Source: CAD feature listing. Evaluate the final solid. Frame: model axes, mm. A direction names the side the tool comes from. Give positions to 0.01 mm unless a question says otherwise; leave off trailing zeros. Order: outer loops, then holes, each group sorted by start corner. A loop starts at its lowest first (then second) coordinate and runs counter-clockwise, first axis right, second up.
1) Section C-C, the plane x = -58. Return loops of the section in (y, z), plus the area to 3 significant figures.
2) Material intervals for line 1 (X direction, y = -17, z = 10.5); line 2 (X direction, y = -42, z = 10); line 3 (Y direction, x = 26, z = 1), sorted ascending.
3) Section A-A, the plane z = 6.35. Give the number of separate pieces and of enclosed holes in the cut face, plus the area to 3 significant figures.
4) Section B-B, the plane y = -6. Return loops of the section in (x, z), plus the area to 3 significant figures.
5) Access query for faces 5 (the face through (-68.885, -16, 6)), 6 (the face through (-62.535, -23, 6)), 7 (the face through (81.585, -43, 6)). Directions: +Z, -Z, +X, -X, +Y, -Y. A direction counts if a zero-diameter tool reaches every point of the face in a straight line with its end or side. Return the directions, or none.
6) First-contact query: P1, Ø6.5, axis at y = -32.5, z = 6, coming from the +X side; P2, Ø4, axis at x = 16, z = 7, coming from the -Y side; P3, Ø4, axis at x = -76, z = 5, coming from the +Y side. Flat tips, straight axial feed; report the tip coordinate or a pass-through.
7) Draft query along X for faces 1 (the face through (-1, 0, 6)), 2 (the face through (76.1, -38.608, 4.8)), 3 (the face through (68.885, -16, 6)), 4 (the face through (73.77, -41.74, 5.74)). Return one class per face: released by +X, released by -X, zero draft, split by the parting line, or undercut.
```python
from build123d import *

# Parameters (mm, degrees)
F1_DEPTH = 12.7
F3_R     = 1.5875
F4_DEPTH = 25.4
F2_R     = 1.5875
F5_DEPTH = 25.4
F6_R     = 2.54
F7_R     = 1.778


with BuildPart() as f1:
    # F0 (on Top) → F1 (new body)
    with BuildSketch(Plane.XY):
        Polygon((-62.5348, 0), (0, 0), (62.5348, 0), (62.5348, -44.958), (81.5848, -44.958), (81.5848, -38.608), (68.8848, -38.608), (68.8848, 0), (68.8848, 6.35), (0, 6.35), (-68.8848, 6.35), (-68.8848, 0), (-68.8848, -38.608), (-81.5848, -38.608), (-81.5848, -44.958), (-62.5348, -44.958), align=None)
    extrude(amount=F1_DEPTH)

    # F3 (on face) → F4 (cut)
    with BuildSketch(Plane(origin=(0, -38.608, 0), x_dir=(-1, 0, 0), z_dir=(0, 1, 0))):
        with Locations((75.2348, 6.35)):
            Circle(F3_R)
    extrude(amount=-F4_DEPTH, mode=Mode.SUBTRACT)

    # F2 (on face) → F5 (cut)
    with BuildSketch(Plane(origin=(0, -38.608, 0), x_dir=(-1, 0, 0), z_dir=(0, 1, 0))):
        with Locations((-75.2348, 6.35)):
            Circle(F2_R)
    extrude(amount=-F5_DEPTH, mode=Mode.SUBTRACT)

    # F6
    f6_edges = [f1.edges().sort_by_distance(p)[0] for p in [
        (81.5848, -38.608, 6.35),
        (68.8848, 6.35, 6.35),
        (68.8848, -38.608, 6.35),
        (-68.8848, 6.35, 6.35),
        (-68.8848, -38.608, 6.35),
        (-81.5848, -38.608, 6.35),
    ]]
    fillet(f6_edges, radius=F6_R)

    # F7
    f7_edges = [f1.edges().sort_by_distance(p)[0] for p in [
        (62.5348, 0, 6.35),
        (-62.5348, 0, 6.35),
        (-62.5348, -44.958, 6.35),
        (62.5348, -44.958, 6.35),
    ]]
    fillet(f7_edges, radius=F7_R)


solid = f1.part
```
From the geometry:
1. outline: (0, 0) - (6.35, 0) - (6.35, 12.7) - (0, 12.7) - close
1. area: 80.6 mm2
2. line 1: x = -68.88 to -62.53, 62.53 to 68.88
2. line 2: x = -81.58 to -62.53, 62.53 to 81.58
2. line 3: y = 0 to 6.35
3. separate pieces: 3
3. enclosed holes: 0
3. area: 1,560 mm2
4. outline: (-68.88, 0) - (-62.53, 0) - (-62.53, 12.7) - (-68.88, 12.7) - close; (62.53, 0) - (68.88, 0) - (68.88, 12.7) - (62.53, 12.7) - close
4. area: 161 mm2
5. face 5: +Z, -Z, -X, +Y
5. face 6: +Z, -Z, -Y
5. face 7: +Z, -Z, +X, +Y, -Y
6. P1: stops at x = 68.88
6. P2: stops at y = 0
6. P3: stops at y = -38.61
7. face 1: undercut
7. face 2: zero draft
7. face 3: released by +X
7. face 4: undercut
